```python
from build123d import *

# Parameters (mm, degrees)
F2_SIZE  = 0.5
F4_DEPTH = 6


with BuildPart() as f1:
    # F0 (on Front) → F1 (revolve)
    with BuildSketch(Plane.XZ):
        Polygon((12.5, 5), (12.5, 7.5), (0, 7.5), (0, 0), (50, 0), (50, 4.25), (49.25, 5), (18.5, 5), (18.375, 4.25), (18.25, 5), align=None)
    revolve(axis=Axis((25, 0, 0), (1, 0, 0)))

    # F2
    f2_edges = [f1.edges().sort_by_distance(p)[0] for p in [
        (0, 0, -7.5),
    ]]
    chamfer(f2_edges, length=F2_SIZE)

    # F3 (on face) → F4 (cut)
    with BuildSketch(Plane(origin=(0, 0, 0), x_dir=(0, -1, 0), z_dir=(-1, 0, 0))):
        Polygon((0, -3.464102), (3, -1.732051), (3, 1.732051), (0, 3.464102), (-3, 1.732051), (-3, -1.732051), align=None)
    extrude(amount=-F4_DEPTH, mode=Mode.SUBTRACT)


solid = f1.part
```
The listing builds one solid part. Answer for the finished solid, in the listing's coordinates (mm). A direction names the side the tool comes from. Round coordinates to 2 decimals unless told otherwise and drop trailing zeros. Write each loop counter-clockwise with the first axis right and the second up, starting at its lowest first coordinate (ties: lowest second). Pieces come first, ordered by that corner, then holes. Notation, with made-up numbers: (45, 30.25) -> (63, 30.25) arc R15 cw to (63, 59.25) -> close; hole circle Ø11 at (17, -15.5). An arc over 180 degrees is marked (long way). Write item = value, one per line.
1) Given pin 1 (2 mm diameter, centred on x = 16, z = -0.5, fed in from -Y); pin 2 (5 mm diameter, centred on x = 9.5, z = -3, fed in from +Y); pin 3 (1.8 mm diameter, centred on y = -1, z = 0, fed in from -X), each flat-ended and moving along its own axis, determine where each tip first touches the part or whether it passes through.
Check values:
pin_1 = -5
pin_2 = 7.48
pin_3 = 6
2) For a pull along Z with two mould halves and no side action, classify faces 1 (the flat face through (6, 0, 0)), 2 (the flat face through (12.5, 5, -2)), 3 (the cylindrical face through (15.33, 4.88, -1.08)) as released by +Z, released by -Z, zero draft, split by the parting line, or undercut.
Check values:
face_1 = undercut
face_2 = zero draft
face_3 = split by the parting line
3) Straight lines are drawn through the part: line 1 along X through (y, z) = (-0.75, -1.75); line 2 along X through (y, z) = (6.5, 0.5); line 3 along Z through (x, y) = (42, -0.25). For each, find the intervals that lie inside material, in ascending order. Write a range as [from, to].
Check values:
line_1 = [6, 50]
line_2 = [0, 12.5]
line_3 = [-4.99, 4.99]
4) Section B-B on x = 35 is taken. Write down the section's boundary in (y, z), plus the area to 3 significant figures.
Check values:
outline = circle Ø10 at (0, 0)
area = 78.5 mm²
5) Section A-A on z = 0 is taken. Write down the section's boundary in (x, y) (3 decimals).
Check values:
outline = (0, -7) -> (0.5, -7.5) -> (12.5, -7.5) -> (12.5, -5) -> (18.25, -5) -> (18.375, -4.25) -> (18.5, -5) -> (49.25, -5) -> (50, -4.25) -> (50, 4.25) -> (49.25, 5) -> (18.5, 5) -> (18.375, 4.25) -> (18.25, 5) -> (12.5, 5) -> (12.5, 7.5) -> (0.5, 7.5) -> (0, 7) -> (0, 3) -> (6, 3) -> (6, -3) -> (0, -3) -> close
6) Which of the six approach directions +Z, -Z, +X, -X, +Y, -Y give full straight-line access (tool end or side, diameter ignored) to faces 4 (the cylindrical face through (33.66, 4.88, -1.08)), 5 (the flat face through (3, -1.5, -2.6)), 6 (the cylindrical face through (6.416, -0.33, -7.493))?
Check values:
face_4 = +X
face_5 = -X
face_6 = +X, -X
7) Section C-C on x = 7.5 is taken. Write down the section's boundary in (y, z).
Check values:
outline = circle Ø15 at (0, 0)
